For this review, use the dimensioned drawing (mm, ordinates from the lowest corner) and the shaded views. A direction names the side the tool comes from. Coordinates: 2 decimals unless noted, no trailing zeros. Order: outer loops, then holes, each group sorted by start corner. A loop starts at its lowest first (then second) coordinate and runs counter-clockwise, first axis right, second up. Notation, with made-up numbers: M -19.5,-7 L 22.5,-7 A31 cw 22.5,31 Z; hole C 80.5,67 d9. An arc over 180 degrees is marked long. Use CSV: the item, a comma, the result in double quotes.
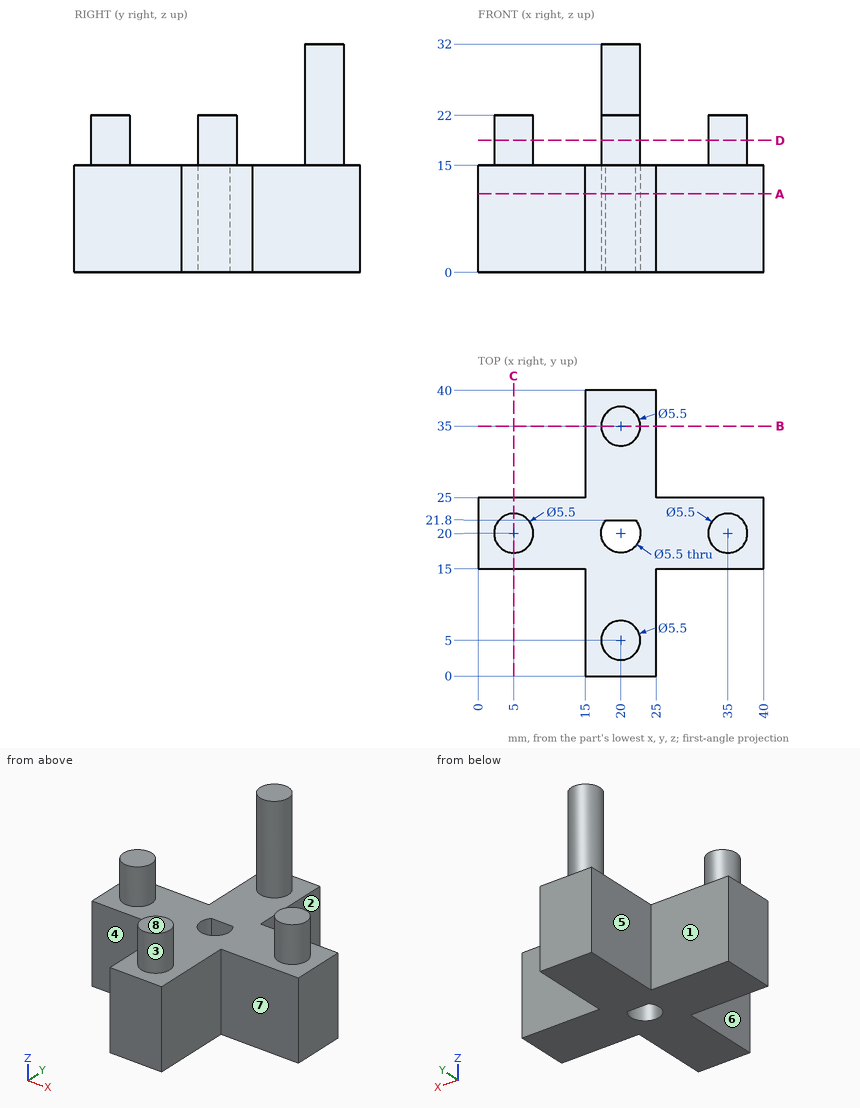
Item 1: Draft analysis for pull direction Y (two halves, no side actions). For the marked faces 1, 2, 3 and 4, state which applies: released by +Y, released by -Y, zero draft, split by the parting line, or undercut.
Solutions:
face 1,"released by +Y"
face 2,"zero draft"
face 3,"undercut"
face 4,"released by -Y"
Item 2: Clearance check with flat-ended pins moving along their axes: pin 1 Ø10 at (x, z) = (9, 15.5) entering from +Y; pin 2 Ø12 at (y, z) = (30.5, 10.5) entering from -X; pin 3 Ø8 at (x, y) = (26.5, 25.5) entering from +Z; pin 4 Ø4.5 at (y, z) = (7, 8) entering from +X. State where each tip first meets the part, or that it passes through.
Solutions:
pin 1,"y = 25"
pin 2,"x = 0"
pin 3,"z = 15"
pin 4,"x = 25"
Item 3: To check wall thickness, follow line 1 along Y through (x, z) = (20, 8); line 2 along X through (y, z) = (20, 8); line 3 along X through (y, z) = (7.5, 13.5). State the ranges of each line that lie inside material, in increasing order. Write a range as [from, to].
Solutions:
line 1,"[0, 17.25], [21.8, 40]"
line 2,"[0, 17.25], [22.75, 40]"
line 3,"[15, 25]"
Item 4: Add section A-A on z = 11. State the section outline as (x, y) points, and give its area (3 significant figures).
Solutions:
outline,"M 0,15 L 15,15 L 15,0 L 25,0 L 25,15 L 40,15 L 40,25 L 25,25 L 25,40 L 15,40 L 15,25 L 0,25 Z; hole M 17.92,21.8 A2.75 ccw long 22.08,21.8 Z"
area,"679 mm^2"
Item 5: Add section B-B on y = 35. State the section outline as (x, z) points.
Solutions:
outline,"M 15,0 L 25,0 L 25,15 L 22.75,15 L 22.75,32 L 17.25,32 L 17.25,15 L 15,15 Z"
Item 6: For the marked faces 5, 6, 7 and 8, list the 3-axis set-ups (+Z, -Z, +X, -X, +Y, -Y) from which the entire face can be reached by the end or side of a thin tool; tool diameter is ignored.
Solutions:
face 5,"+Z, -Z, -X, +Y"
face 6,"+Z, -Z, -X, -Y"
face 7,"+Z, -Z, +X, -Y"
face 8,"+Z, +X, -X, -Y"
Item 7: Add section D-D on z = 18.5. State the section outline as (x, y) points, and give its area (3 significant figures).
Solutions:
outline,"C 5,20 d5.5; C 20,5 d5.5; C 20,35 d5.5; C 35,20 d5.5"
area,"95.0 mm^2"
Item 8: Add section C-C on x = 5. State the section outline as (y, z) points, and give its area (4 significant figures).
Solutions:
outline,"M 15,0 L 25,0 L 25,15 L 22.75,15 L 22.75,22 L 17.25,22 L 17.25,15 L 15,15 Z"
area,"188.5 mm^2"
